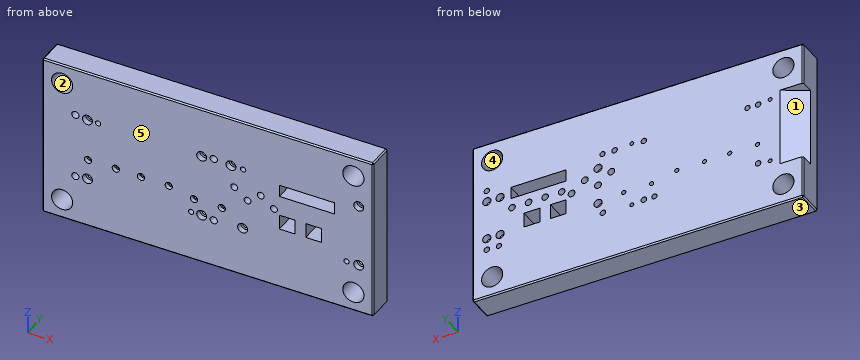
```python
from build123d import *

# Parameters (mm, degrees)
SKETCH1_W                                           = 500
SKETCH1_H                                           = 250
BOSS_EXTRUDE1_DEPTH                                 = 40
F_32_0_32_DIAMETER_HOLE1_D                          = 32
CHAMFER1_SIZE                                       = 2
CBORE_FOR_M8_HEX_SOCKET_HEAD_CAP_SCREW1_D           = 8.4
CBORE_FOR_M8_HEX_SOCKET_HEAD_CAP_SCREW1_CBORE_D     = 15
CBORE_FOR_M8_HEX_SOCKET_HEAD_CAP_SCREW1_CBORE_DEPTH = 8.6
F_8_0MM_DOWEL_HOLE1_D                               = 8
SKETCH16_R                                          = 6.25
SKETCH16_R_2                                        = 5
CUT_EXTRUDE1_DEPTH                                  = 10
CUT_EXTRUDE2_REACH                                  = 284.356
SKETCH18_R                                          = 3
SKETCH19_R                                          = 5.5
CUT_EXTRUDE3_DEPTH                                  = 33
CBORE_FOR_M6_HEX_SOCKET_HEAD_CAP_SCREW1_D           = 6.4
CBORE_FOR_M6_HEX_SOCKET_HEAD_CAP_SCREW1_CBORE_D     = 11
CBORE_FOR_M6_HEX_SOCKET_HEAD_CAP_SCREW1_CBORE_DEPTH = 6.4
CUT_EXTRUDE4_REACH                                  = 284.356
SKETCH23_R                                          = 5.174550649
SKETCH23_W                                          = 83.404692778
SKETCH23_H                                          = 18.284692778
SKETCH23_W_2                                        = 23.904692778
SKETCH23_H_2                                        = 22.564692778
SKETCH23_W_3                                        = 23.654692778


with BuildPart() as part:
    # Sketch1 → Boss-Extrude1 (new body)
    with BuildSketch(Plane(origin=(0, 0, 0), x_dir=(1, 0, 0), z_dir=(0, 1, 0))):
        Rectangle(SKETCH1_W, SKETCH1_H)
    extrude(amount=-BOSS_EXTRUDE1_DEPTH)

    # Ø32.0 (32) Diameter Hole1 (through all)
    with Locations(Plane(origin=(0, 0, 0), x_dir=(1, 0, 0), z_dir=(0, 1, 0))):
        with Locations((-220, 95), (-220, -95), (220, -95), (220, 95)):
            Hole(F_32_0_32_DIAMETER_HOLE1_D / 2)

    # Chamfer1
    chamfer1_edges = [part.edges().sort_by_distance(p)[0] for p in [
        (-250, -40, 0),
        (0, -40, 125),
        (250, -40, 0),
        (0, 0, 125),
        (-250, 0, 0),
        (0, 0, -125),
        (250, 0, 0),
        (250, -20, 125),
        (-250, -20, 125),
        (-250, -20, -125),
        (250, -20, -125),
        (0, -40, -125),
    ]]
    chamfer(chamfer1_edges, length=CHAMFER1_SIZE)

    # CBORE for M8 Hex Socket Head Cap Screw1 (through all)
    with Locations(Plane(origin=(0, -40, 0), x_dir=(-1, 0, 0), z_dir=(0, -1, 0))):
        with Locations((-228, 48), (-52.632503002, 48), (-228, -48), (-35, -48), (9.219, 48), (181.75, 48), (181.75, -48), (9.219, -48)):
            CounterBoreHole(CBORE_FOR_M8_HEX_SOCKET_HEAD_CAP_SCREW1_D / 2, CBORE_FOR_M8_HEX_SOCKET_HEAD_CAP_SCREW1_CBORE_D / 2, CBORE_FOR_M8_HEX_SOCKET_HEAD_CAP_SCREW1_CBORE_DEPTH)

    # Ø8.0mm Dowel Hole1 (through all)
    with Locations(Plane(origin=(0, -40, 0), x_dir=(-1, 0, 0), z_dir=(0, -1, 0))):
        with Locations((-53.4, -48), (-209.6, 48), (25.219, 48), (165.75, -48)):
            Hole(F_8_0MM_DOWEL_HOLE1_D / 2)

    # Sketch16 → Cut-Extrude1 (cut)
    with BuildSketch(Plane(origin=(0, 0, 0), x_dir=(1, 0, 0), z_dir=(0, 1, 0))):
        with Locations(Location((60, 30, 0), (0, 0, 270))):
            Circle(SKETCH16_R)
        with Locations(Location((208, 30, 0), (0, 0, 270))):
            Circle(SKETCH16_R)
        with Locations(Location((228, 30, 0), (0, 0, 270))):
            Circle(SKETCH16_R)
        with Locations(Location((228, -30.5, 0), (0, 0, 270))):
            Circle(SKETCH16_R)
        with Locations(Location((208, -30.5, 0), (0, 0, 270))):
            Circle(SKETCH16_R)
        with Locations(Location((190, -7.72, 0), (0, 0, 270))):
            Circle(SKETCH16_R_2)
        with Locations(Location((165, -7.72, 0), (0, 0, 270))):
            Circle(SKETCH16_R_2)
        with Locations(Location((140, -7.72, 0), (0, 0, 270))):
            Circle(SKETCH16_R_2)
        with Locations(Location((115, -7.72, 0), (0, 0, 270))):
            Circle(SKETCH16_R_2)
        with Locations(Location((60, -27.22, 0), (0, 0, 270))):
            Circle(SKETCH16_R)
    extrude(amount=-CUT_EXTRUDE1_DEPTH, mode=Mode.SUBTRACT)

    # Sketch18 → Cut-Extrude2 (cut, up to next)
    with BuildSketch(Plane(origin=(0, 0, 0), x_dir=(1, 0, 0), z_dir=(0, 1, 0)), mode=Mode.PRIVATE) as cut_extrude2_sk1:
        with Locations(Location((-200, -50, 0), (0, 0, 270))):
            Circle(SKETCH18_R)
    cut_extrude2_tool1 = extrude(cut_extrude2_sk1.sketch, amount=-CUT_EXTRUDE2_REACH, mode=Mode.PRIVATE) & part.part
    # Sketch18 → Cut-Extrude2 (cut, up to next)
    with BuildSketch(Plane(origin=(0, 0, 0), x_dir=(1, 0, 0), z_dir=(0, 1, 0)), mode=Mode.PRIVATE) as cut_extrude2_sk2:
        with Locations(Location((-200, 50, 0), (0, 0, 270))):
            Circle(SKETCH18_R)
    cut_extrude2_tool2 = extrude(cut_extrude2_sk2.sketch, amount=-CUT_EXTRUDE2_REACH, mode=Mode.PRIVATE) & part.part
    # Sketch18 → Cut-Extrude2 (cut, up to next)
    with BuildSketch(Plane(origin=(0, 0, 0), x_dir=(1, 0, 0), z_dir=(0, 1, 0)), mode=Mode.PRIVATE) as cut_extrude2_sk3:
        with Locations(Location((9.031, 50, 0), (0, 0, 270))):
            Circle(SKETCH18_R)
    cut_extrude2_tool3 = extrude(cut_extrude2_sk3.sketch, amount=-CUT_EXTRUDE2_REACH, mode=Mode.PRIVATE) & part.part
    # Sketch18 → Cut-Extrude2 (cut, up to next)
    with BuildSketch(Plane(origin=(0, 0, 0), x_dir=(1, 0, 0), z_dir=(0, 1, 0)), mode=Mode.PRIVATE) as cut_extrude2_sk4:
        with Locations(Location((9.031, -50, 0), (0, 0, 270))):
            Circle(SKETCH18_R)
    cut_extrude2_tool4 = extrude(cut_extrude2_sk4.sketch, amount=-CUT_EXTRUDE2_REACH, mode=Mode.PRIVATE) & part.part
    add(cut_extrude2_tool1.solids().sort_by_distance((-200, 0, 50))[0], mode=Mode.SUBTRACT)
    add(cut_extrude2_tool2.solids().sort_by_distance((-200, 0, -50))[0], mode=Mode.SUBTRACT)
    add(cut_extrude2_tool3.solids().sort_by_distance((9.031, 0, -50))[0], mode=Mode.SUBTRACT)
    add(cut_extrude2_tool4.solids().sort_by_distance((9.031, 0, 50))[0], mode=Mode.SUBTRACT)

    # Sketch19 → Cut-Extrude3 (cut)
    with BuildSketch(Plane.XZ.offset(40)):
        with Locations(Location((-200, 50, 0), (0, 0, 270))):
            Circle(SKETCH19_R)
        with Locations(Location((-200, -50, 0), (0, 0, 270))):
            Circle(SKETCH19_R)
        with Locations(Location((9.031, -50, 0), (0, 0, 270))):
            Circle(SKETCH19_R)
        with Locations(Location((9.031, 50, 0), (0, 0, 270))):
            Circle(SKETCH19_R)
    extrude(amount=-CUT_EXTRUDE3_DEPTH, mode=Mode.SUBTRACT)

    # CBORE for M6 Hex Socket Head Cap Screw1 (through all)
    with Locations(Plane(origin=(0, -40, 0), x_dir=(-1, 0, 0), z_dir=(0, -1, 0))):
        with Locations((-21.125, 25.691000385), (20.875, 25.691000385), (58.875, 17.152366083), (100.875, 17.152366083), (138.875, 16.78), (180.875, 16.78)):
            CounterBoreHole(CBORE_FOR_M6_HEX_SOCKET_HEAD_CAP_SCREW1_D / 2, CBORE_FOR_M6_HEX_SOCKET_HEAD_CAP_SCREW1_CBORE_D / 2, CBORE_FOR_M6_HEX_SOCKET_HEAD_CAP_SCREW1_CBORE_DEPTH)

    # Sketch23 → Cut-Extrude4 (cut, up to next)
    with BuildSketch(Plane.XZ.offset(40), mode=Mode.PRIVATE) as cut_extrude4_sk1:
        with Locations(Location((100, -0.28, 0), (0, 0, 270))):
            Circle(SKETCH23_R)
    cut_extrude4_tool1 = extrude(cut_extrude4_sk1.sketch, amount=-CUT_EXTRUDE4_REACH, mode=Mode.PRIVATE) & part.part
    # Sketch23 → Cut-Extrude4 (cut, up to next)
    with BuildSketch(Plane.XZ.offset(40), mode=Mode.PRIVATE) as cut_extrude4_sk2:
        with Locations(Location((80, 14.72, 0), (0, 0, 270))):
            Circle(SKETCH23_R)
    cut_extrude4_tool2 = extrude(cut_extrude4_sk2.sketch, amount=-CUT_EXTRUDE4_REACH, mode=Mode.PRIVATE) & part.part
    # Sketch23 → Cut-Extrude4 (cut, up to next)
    with BuildSketch(Plane.XZ.offset(40), mode=Mode.PRIVATE) as cut_extrude4_sk3:
        with Locations(Location((60, -0.28, 0), (0, 0, 270))):
            Circle(SKETCH23_R)
    cut_extrude4_tool3 = extrude(cut_extrude4_sk3.sketch, amount=-CUT_EXTRUDE4_REACH, mode=Mode.PRIVATE) & part.part
    # Sketch23 → Cut-Extrude4 (cut, up to next)
    with BuildSketch(Plane.XZ.offset(40), mode=Mode.PRIVATE) as cut_extrude4_sk4:
        with Locations(Location((40, 14.72, 0), (0, 0, 270))):
            Circle(SKETCH23_R)
    cut_extrude4_tool4 = extrude(cut_extrude4_sk4.sketch, amount=-CUT_EXTRUDE4_REACH, mode=Mode.PRIVATE) & part.part
    # Sketch23 → Cut-Extrude4 (cut, up to next)
    with BuildSketch(Plane.XZ.offset(40), mode=Mode.PRIVATE) as cut_extrude4_sk5:
        with Locations((150, 32.16)):
            Rectangle(SKETCH23_W, SKETCH23_H)
    cut_extrude4_tool5 = extrude(cut_extrude4_sk5.sketch, amount=-CUT_EXTRUDE4_REACH, mode=Mode.PRIVATE) & part.part
    # Sketch23 → Cut-Extrude4 (cut, up to next)
    with BuildSketch(Plane.XZ.offset(40), mode=Mode.PRIVATE) as cut_extrude4_sk6:
        with Locations((160, -18.86)):
            Rectangle(SKETCH23_W_2, SKETCH23_H_2)
    cut_extrude4_tool6 = extrude(cut_extrude4_sk6.sketch, amount=-CUT_EXTRUDE4_REACH, mode=Mode.PRIVATE) & part.part
    # Sketch23 → Cut-Extrude4 (cut, up to next)
    with BuildSketch(Plane.XZ.offset(40), mode=Mode.PRIVATE) as cut_extrude4_sk7:
        with Locations((120.125, -18.86)):
            Rectangle(SKETCH23_W_3, SKETCH23_H_2)
    cut_extrude4_tool7 = extrude(cut_extrude4_sk7.sketch, amount=-CUT_EXTRUDE4_REACH, mode=Mode.PRIVATE) & part.part
    add(cut_extrude4_tool1.solids().sort_by_distance((100, -40, -0.28))[0], mode=Mode.SUBTRACT)
    add(cut_extrude4_tool2.solids().sort_by_distance((80, -40, 14.72))[0], mode=Mode.SUBTRACT)
    add(cut_extrude4_tool3.solids().sort_by_distance((60, -40, -0.28))[0], mode=Mode.SUBTRACT)
    add(cut_extrude4_tool4.solids().sort_by_distance((40, -40, 14.72))[0], mode=Mode.SUBTRACT)
    add(cut_extrude4_tool5.solids().sort_by_distance((150, -40, 32.16))[0], mode=Mode.SUBTRACT)
    add(cut_extrude4_tool6.solids().sort_by_distance((160, -40, -18.86))[0], mode=Mode.SUBTRACT)
    add(cut_extrude4_tool7.solids().sort_by_distance((120.125, -40, -18.86))[0], mode=Mode.SUBTRACT)

    # Cut-Sweep1: sweep along a path in Sketch24
    with BuildLine(Plane(origin=(0, 0, 0), x_dir=(1, 0, 0), z_dir=(0, 1, 0))) as cut_sweep1_path:
        Line((-215, -60), (-215, 60))
    # Sketch25 → Cut-Sweep1 (sweep, cut)
    with BuildSketch(Plane.XY):
        Polygon((-215, 0), (-250, -20.207259422), (-250, 0), align=None)
    sweep(path=cut_sweep1_path.line, mode=Mode.SUBTRACT)


solid = part.part
```
The listing builds one solid part. Answer for the finished solid, in the listing's coordinates (mm). Face numbers are marked on the shaded views. A direction names the side the tool comes from. Coordinates: 2 decimals unless noted, no trailing zeros. Write each loop counter-clockwise with the first axis right and the second up, starting at its lowest first coordinate (ties: lowest second). Pieces come first, ordered by that corner, then holes.
Q1. The mould has two halves that part along Z. Classify the marked faces 3, 4 and 5: released by +Z, released by -Z, zero draft, split by the parting line, or undercut.
Returned:
face 3: released by -Z
face 4: undercut
face 5: zero draft
Q2. Which of the six approach directions +Z, -Z, +X, -X, +Y, -Y give full straight-line access (tool end or side, diameter ignored) to the marked faces 1 and 2?
Returned:
face 1: -X, +Y
face 2: +Y, -Y
Q3. Find the intervals of material crossed by line 1 along X through (y, z) = (-22, -95); line 2 along Z through (x, y) = (123.5, -34.5); line 3 along Z through (x, y) = (-10.5, -17), in increasing order.
Returned:
line 1: x = -250 to -236, -204 to 204, 236 to 250
line 2: z = -125 to -30.14, -7.58 to 23.02, 41.3 to 125
line 3: z = -125 to -52, -44 to 44, 52 to 125
Q4. Given P1, Ø7.5, axis at x = -181.75, z = -48, coming from the -Y side; P2, Ø8, axis at x = 190, z = 7, coming from the +Y side, each flat-ended and moving along its own axis, determine where each tip first touches the part or whether it passes through.
Returned:
P1: passes through
P2: stops at y = -10
Q5. Section C-C, the plane x = 165 is taken. Write down the section's boundary in (y, z).
Returned:
outline: (-40, -123) - (-38, -125) - (-2, -125) - (0, -123) - (0, -30.14) - (-40, -30.14) - close; (-40, -7.58) - (0, -7.58) - (0, 2.72) - (-10, 2.72) - (-10, 12.72) - (0, 12.72) - (0, 23.02) - (-40, 23.02) - close; (-40, 41.3) - (0, 41.3) - (0, 123) - (-2, 125) - (-38, 125) - (-40, 123) - close
Q6. Section A-A, the plane z = 95 is taken. Write down the section's boundary in (x, y).
Returned:
outline: (-250, -38) - (-248, -40) - (-236, -40) - (-236, 0) - (-248, 0) - (-250, -2) - close; (-204, -40) - (204, -40) - (204, 0) - (-204, 0) - close; (236, -40) - (248, -40) - (250, -38) - (250, -2) - (248, 0) - (236, 0) - close
Q7. Section B-B, the plane x = 100 is taken. Write down the section's boundary in (y, z).
Returned:
outline: (-40, -123) - (-38, -125) - (-2, -125) - (0, -123) - (0, -5.45) - (-40, -5.45) - close; (-40, 4.89) - (0, 4.89) - (0, 123) - (-2, 125) - (-38, 125) - (-40, 123) - close
Q8. Section D-D, the plane y = -26 is taken. Give the number of separate pieces and of enclosed holes in the cut face, then the cut area to 3 significant figures.
Returned:
separate pieces: 1
enclosed holes: 33
area: 118,000 mm2
